Autodesk Inventor part; units mm, degrees
ref_plane "YZ Plane" through (0, 0, 0) normal (1, 0, 0) x (0, 1, 0)
ref_plane "XZ Plane" through (0, 0, 0) normal (0, 1, 0) x (-1, 0, 0)
ref_plane "XY Plane" through (0, 0, 0) normal (0, 0, 1) x (1, 0, 0)
sketch "Sketch1" plane through (0, 0, 0) normal (0, 0, 1) x (1, 0, 0)
  circle A0 centre (0, 0) radius 17.4793 construction
  circle A1 centre (0, 0) radius 23.2285 construction
  circle A2 centre (0, 0) radius 6.35
  circle A3 centre (0, 0) radius 2.5019
  dimension "d0" = 46.4569
  dimension "d1" = 34.9586
  dimension "d2" = 12.7
  dimension "d3" = 5.0038
extrude "Extrusion1" add sketch "Sketch1" along normal blind 27.8384
sketch "Sketch2" plane through (0, 0, 0) normal (1, 0, 0) x (0, 1, 0)
  line L0 (0, 0) -> (0, 27.8384) construction
  line L1 (6.35, 27.8384) -> (-6.35, 27.8384) construction
  circle A0 centre (0, 13.9192) radius 2.65
  dimension "d6" = 5.3
extrude "Extrusion2" cut sketch "Sketch2" against normal through all
ref_plane "Work Plane1" through (0, 0, 0) normal (0, 0, 1) x (1, 0, 0)
sketch "Sketch3" plane through (0, 0, 0) normal (0, 0, 1) x (1, 0, 0)
  circle A0 centre (0, 0) radius 22.9615 construction
properties part number "Inner Gear Extruded"
Part model, mm, in its own coordinate system. Coordinates: 2 decimals unless noted, no trailing zeros. Order: outer loops, then holes, each group sorted by start corner. A loop starts at its lowest first (then second) coordinate and runs counter-clockwise, first axis right, second up. Notation, with made-up numbers: M -31.75,78 L 16.25,78 A27 ccw 16.25,102 Z; hole C -9,59 d1. An arc over 180 degrees is marked long. One line per question, with ' | ' between items.
Q1. Drill centre lines: line 1 (Y direction, x = 1.25, z = 17.5); line 2 (X direction, y = 5, z = 1.5); line 3 (X direction, y = -4, z = 25.5). Where is each one in solid material? Low to high.
A:
line 1: y = -6.23 to -2.17, 2.17 to 6.23 | line 2: x = -3.91 to 3.91 | line 3: x = -4.93 to 4.93
Q2. Slice it at A-A (y = 0). Give the cut face in (x, z), and give its area (3 significant figures).
A:
outline: M -6.35,0 L -2.5,0 L -2.5,11.27 L -6.35,11.27 Z; M -6.35,16.57 L -2.5,16.57 L -2.5,27.84 L -6.35,27.84 Z; M 2.5,0 L 6.35,0 L 6.35,27.84 L 2.5,27.84 Z | area: 194 mm^2
Q3. Pin check, flat tips, straight feed: P1, Ø1, axis at x = 3.5, z = 16, coming from the +Y side; P2, Ø1, axis at y = -3.5, z = 8, coming from the -X side; P3, Ø2, axis at y = 2, z = 20.5, coming from the -X side. Stop position of each tip, or through.
A:
P1: stops at y = 5.6 | P2: stops at x = -5.6 | P3: stops at x = -6.27
Q4. Slice it at B-B (z = 4.5). Give the cut face in (x, y).
A:
outline: C 0,0 d12.7; hole C 0,0 d5
Q5. Two-plate mould, pull along Y, no slides. Class faces 1 (the face through (2.31, 0.96, 13.72)), 2 (the face through (3, 0, 0)), 3 (the face through (6.057, -1.907, 13.724)), 4 (the face through (-3.836, -1.953, 15.71)): +Y half, -Y half, draft (parallel to the pull), parting line (faces both ways), or undercut.
A:
face 1: undercut | face 2: draft | face 3: parting line | face 4: undercut
Q6. Slice it at C-C (x = 1). Give the cut face in (y, z).
A:
outline: M -6.27,0 L -2.29,0 L -2.29,27.84 L -6.27,27.84 Z; M 2.29,0 L 6.27,0 L 6.27,27.84 L 2.29,27.84 Z
Q7. Slice it at D-D (x = -3.25). Give the cut face in (y, z), and give its area (3 significant figures).
A:
outline: M -5.46,0 L 5.46,0 L 5.46,27.84 L -5.46,27.84 Z; hole C 0,13.92 d5.3 | area: 282 mm^2
